```python
from build123d import *

# Parameters (mm, degrees)
SKETCH2_W             = 17.554431489
SKETCH2_H             = 1.95
BOSS_EXTRUDE1_DEPTH   = 8.75
BOSS_EXTRUDE1_2_DEPTH = 8.75
CUT_EXTRUDE1_DEPTH    = 26.518349076
SKETCH4_W             = 22.027215745
SKETCH4_H             = 12.505427167
BOSS_EXTRUDE2_DEPTH   = 30
SKETCH5_R             = 1.5
CUT_EXTRUDE2_DEPTH    = 12
SKETCH6_W             = 22.027215745
SKETCH6_H             = 12.505427167
SKETCH6_W_2           = 17.554431489
SKETCH6_H_2           = 1.95
CUT_EXTRUDE3_DEPTH    = 2.5
SKETCH7_R             = 1.5
CUT_EXTRUDE4_DEPTH    = 13
SKETCH8_R             = 1.5
CUT_EXTRUDE5_DEPTH    = 28
FILLET3_R             = 1
SKETCH9_W             = 22.02721574
SKETCH9_H             = 2
CUT_EXTRUDE6_DEPTH    = 11


with BuildPart() as part:
    # Sketch2 → Boss-Extrude1 (new body)
    with BuildSketch(Plane.XY):
        with Locations((-13.228930986, -27.845183414)):
            Rectangle(SKETCH2_W, SKETCH2_H)
    extrude(amount=BOSS_EXTRUDE1_DEPTH)


with BuildPart() as body_2:
    # Sketch2 → Boss-Extrude1 2 (new body)
    with BuildSketch(Plane.XY):
        with Locations((-13.228930986, -20.289756247)):
            Rectangle(SKETCH2_W, SKETCH2_H)
    extrude(amount=BOSS_EXTRUDE1_2_DEPTH)


with BuildPart() as cut_extrude1_tool:
    # Sketch3 → Cut-Extrude1 (new, through all)
    with BuildSketch(Plane(origin=(0, -19.314756247, 0), x_dir=(1, 0, 0), z_dir=(0, 1, 0))):
        with BuildLine():
            ThreePointArc((-13.228930986, -8.75), (-7.041746651, -6.187184335), (-4.478930986, 0))
            add(Edge.make_bspline(
                [(-4.478930986, 0), (1.138349918, -4.151657709), (-4.451715242, -8.75)],
                knots=[0, 0, 0, 1, 1, 1], degree=2))
            add(Edge.make_bspline(
                [(-22.006146731, -8.75), (-13.228930986, -12.473510392), (-4.451715242, -8.75)],
                knots=[0, 0, 0, 1, 1, 1], degree=2))
            add(Edge.make_bspline(
                [(-21.978930986, 0), (-25.926969228, -4.242865138), (-22.006146731, -8.75)],
                knots=[0, 0, 0, 1, 1, 1], degree=2))
            ThreePointArc((-21.978930986, 0), (-19.416115322, -6.187184335), (-13.228930986, -8.75))
        make_face()
    extrude(amount=-CUT_EXTRUDE1_DEPTH)


with BuildPart() as part_1:
    add(part.part)

    # Cut-Extrude1: cut by cut_extrude1_tool
    add(cut_extrude1_tool.part, mode=Mode.SUBTRACT)



with BuildPart() as body_2_1:
    add(body_2.part)

    # Cut-Extrude1: cut by cut_extrude1_tool
    add(cut_extrude1_tool.part, mode=Mode.SUBTRACT)


with BuildPart() as part_2:
    add(part_1.part)

    add(body_2_1.part)  # Boss-Extrude2 merges body 2
    # Sketch4 → Boss-Extrude2 (add)
    with BuildSketch(Plane(origin=(0, 0, 0), x_dir=(-1, 0, 0), z_dir=(0, 0, -1))):
        with Locations((13.242538859, -24.067469831)):
            Rectangle(SKETCH4_W, SKETCH4_H)
    extrude(amount=BOSS_EXTRUDE2_DEPTH)

    # Sketch5 → Cut-Extrude2 (cut)
    with BuildSketch(Plane(origin=(0, -19.314756247, 0), x_dir=(1, 0, 0), z_dir=(0, 1, 0))):
        with Locations(Location((-13.228930986, -2.25, 0), (0, 0, 270))):
            Circle(SKETCH5_R)
    extrude(amount=-CUT_EXTRUDE2_DEPTH, mode=Mode.SUBTRACT)

    # Sketch6 → Cut-Extrude3 (cut)
    with BuildSketch(Plane.XY):
        with Locations((-13.242538859, -24.067469831)):
            Rectangle(SKETCH6_W, SKETCH6_H)
        with Locations((-13.228930986, -27.845183414)):
            Rectangle(SKETCH6_W_2, SKETCH6_H_2, mode=Mode.SUBTRACT)
        with Locations((-13.228930986, -20.289756247)):
            Rectangle(SKETCH6_W_2, SKETCH6_H_2, mode=Mode.SUBTRACT)
    extrude(amount=-CUT_EXTRUDE3_DEPTH, mode=Mode.SUBTRACT)

    # Sketch7 → Cut-Extrude4 (cut)
    with BuildSketch(Plane(origin=(0, -17.814756247, 0), x_dir=(1, 0, 0), z_dir=(0, 1, 0))):
        with Locations(Location((-13.242538859, 23.405672985, 0), (0, 0, 270))):
            Circle(SKETCH7_R)
        with BuildLine():
            Line((-22.086865874, 21.155672985), (-24.256146731, 21.155672985))
            add(Edge.make_bspline(
                [(-2.228930986, 21.155672985), (11.471530889, 27.189710441), (-11.765166974, 53.431279988), (-37.007876173, 21.523583672), (-24.256146731, 21.155672985)],
                knots=[0, 0, 0, 0, 0.52011282, 1, 1, 1, 1], degree=3))
            add(Edge.make_bspline(
                [(-5.046294073, 28.201654423), (-2.731488374, 25.068620188), (-2.228930986, 21.155672985)],
                knots=[0, 0, 0, 1, 1, 1], degree=2))
            Line((-5.046294073, 28.201654423), (-13.242538859, 30))
            ThreePointArc((-13.242538859, 30), (-19.496422466, 27.409556592), (-22.086865874, 21.155672985))
        make_face()
    extrude(amount=-CUT_EXTRUDE4_DEPTH, mode=Mode.SUBTRACT)

    # Sketch8 → Cut-Extrude5 (cut)
    with BuildSketch(Plane.XY.offset(-2.5)):
        with Locations((-18.011106811, -24.06746983)):
            Circle(SKETCH8_R)
        with Locations((-8.473970906, -24.06746983)):
            Circle(SKETCH8_R)
    extrude(amount=-CUT_EXTRUDE5_DEPTH, mode=Mode.SUBTRACT)

    # Fillet3
    fillet3_edges = [part_2.edges().sort_by_distance(p)[0] for p in [
        (-24.256146731, -24.06746983, -2.5),
        (-24.256146731, -24.06746983, -21.155672985),
        (-2.228930986, -24.06746983, -2.5),
        (-5.046294073, -24.06746983, -28.201654423),
    ]]
    fillet(fillet3_edges, radius=FILLET3_R)

    # Sketch9 → Cut-Extrude6 (cut)
    with BuildSketch(Plane.XY.offset(-32.5)):
        with Locations((-13.24253886, -20.31475625)):
            Rectangle(SKETCH9_W, SKETCH9_H)
        with Locations((-13.24253886, -27.836055834)):
            Rectangle(SKETCH9_W, SKETCH9_H)
    extrude(amount=CUT_EXTRUDE6_DEPTH, mode=Mode.SUBTRACT)


solid = part_2.part
```
Input: part model. Units: mm. Frame: model coordinates. A direction names the side the tool comes from. Round coordinates to 2 decimals unless told otherwise and drop trailing zeros. Order: outer loops, then holes, each group sorted by start corner. A loop starts at its lowest first (then second) coordinate and runs counter-clockwise, first axis right, second up. Notation, with made-up numbers: (82.5, 64.25) - (93.5, 64.25) arc R14 cw to (93.5, 82.25) - close; hole circle Ø10 at (-12.5, -37.5). An arc over 180 degrees is marked (long way). One line per question, with ' | ' between items. Start each with the question number.
1) Ray query, probe 1 along Y at (x, z) = (-20.25, -23); probe 2 along Z at (x, y) = (-13.25, -20.25); probe 3 along Y at (x, z) = (-18.75, 5). Return the intervals inside material, ascending.
2) Cut plane B-B, the plane x = -18.75. Return the cut outline in (y, z).
3) Cut plane A-A, the plane z = 2.25. Return the cut outline in (x, y).
4) Contact query for flat-ended pins moving along their axis: P1, Ø5, axis at x = -7, y = -23, coming from the -Z side; P2, Ø4, axis at x = -7.5, y = -24, coming from the -Z side; P3, Ø4, axis at x = -13.23, z = 2.25, coming from the -Y side; P4, Ø1.8, axis at x = -13.24, z = -23.41, coming from the +Y side. Output: stop coordinate, or through.
5) Pull-direction query (Y, two-part tool) for faces 1 (the flat face through (-12, -26.836, -25)), 2 (the cylindrical face through (-23.96, -23.98, -2.79)), 3 (the flat face through (-13, -24, -2.5)), 4 (the flat face through (-13, -17.815, -16)); classes: +Y half, -Y half, draft (parallel to the pull), parting line (faces both ways), or undercut.
6) Set-up query: faces 5 (the cylindrical face through (-12.792, -29.568, -21.975)), 6 (the flat face through (-9.28, -29.57, -29.13)), 7 (the flat face through (-22.006, -28, -1)), 8 (the flat face through (-12, -21.315, -25)), 9 (the flat face through (-4.452, -28, -1)). Return all of +Z, -Z, +X, -X, +Y, -Y with unobstructed straight access to the full face (end or side cutting, diameter ignored); none if empty.
7) Cut plane D-D, the plane z = -13.5. Return the cut outline in (x, y).
8) Cut plane C-C, the plane x = -12.75. Give the number of separate pieces and of enclosed holes in the cut face, then the cut area to 3 significant figures.
Worked out:
1) probe 1: y = -30.32 to -28.84, -26.84 to -21.31, -19.31 to -17.81 | probe 2: z = -21.5 to 0.75, 3.75 to 8.75 | probe 3: y = -28.82 to -26.87, -21.26 to -19.31
2) outline: (-30.32, -28.08) - (-28.84, -28.08) - (-28.84, -21.5) - (-26.84, -21.5) - (-26.84, -28.08) - (-25.37, -28.08) - (-25.37, -2.5) - (-26.87, -2.5) - (-26.87, 6.79) - (-28.82, 6.79) - (-28.82, -2.5) - (-30.32, -2.5) - close; (-22.76, -28.08) - (-21.31, -28.08) - (-21.31, -21.5) - (-19.31, -21.5) - (-19.31, -28.08) - (-17.81, -28.08) - (-17.81, -2.5) - (-19.31, -2.5) - (-19.31, 6.79) - (-21.26, 6.79) - (-21.26, -2.5) - (-22.76, -2.5) - close
3) outline: (-21.68, -28.82) - (-14.73, -28.82) - (-14.73, -26.87) - (-21.68, -26.87) - close; (-21.68, -21.26) - (-14.73, -21.26) - (-14.73, -19.31) - (-21.68, -19.31) - close; (-11.73, -28.82) - (-4.77, -28.82) - (-4.77, -26.87) - (-11.73, -26.87) - close; (-11.73, -21.26) - (-4.77, -21.26) - (-4.77, -19.31) - (-11.73, -19.31) - close
4) P1: stops at z = -29.18 | P2: stops at z = -29.06 | P3: stops at y = -28.82 | P4: passes through
5) face 1: undercut | face 2: draft | face 3: undercut | face 4: +Y half
6) face 5: +Y, -Y | face 6: -Z, +X, +Y, -Y | face 7: +Z, -X, +Y, -Y | face 8: -Z, +X, -X | face 9: +Z, +X, +Y, -Y
7) outline: (-24.26, -30.32) - (-2.23, -30.32) - (-2.23, -17.81) - (-24.26, -17.81) - close; hole circle Ø3 at (-18.01, -24.07); hole circle Ø3 at (-8.47, -24.07)
8) separate pieces: 6 | enclosed holes: 0 | area: 318 mm^2
